Geometry: see drawing. Coordinates: mm, zero at the bounding-box minimum. Round coordinates to 2 decimals unless told otherwise and drop trailing zeros. Loops run counter-clockwise (first coordinate to the right, second up) from the corner with the lowest first, then second, coordinate; pieces in that order, holes last.
(1) Line query: line 1 (Y direction, x = 40, z = 2.25); line 2 (Y direction, x = 52, z = 0.35); line 3 (X direction, y = 85, z = 2.4). Output: solid intervals per line, ascending.
(2) Cut plane A-A, the plane y = 155. Output: boundary loops of the cut face in (x, z), and give its area (3 significant figures).
(3) Cut plane D-D, the plane y = 133.5. Output: boundary loops of the cut face in (x, z), and give its area (3 significant figures).
(4) Cut plane C-C, the plane z = 1.5. Output: boundary loops of the cut face in (x, y), and give its area (3 significant figures).
(5) Cut plane B-B, the plane x = 40. Output: boundary loops of the cut face in (y, z), and give its area (3 significant figures).
(6) First-contact query: pin 1 Ø10 at (x, y) = (21.5, 147.5) entering from -Z; pin 2 Ø2 at (x, z) = (14.5, 2.5) entering from +Y; pin 3 Ø1.5 at (y, z) = (37.5, 2.5) entering from +X; pin 4 Ø2.5 at (y, z) = (130.5, 3.5) entering from -X. Flat tips, straight axial feed; report the tip coordinate or a pass-through.
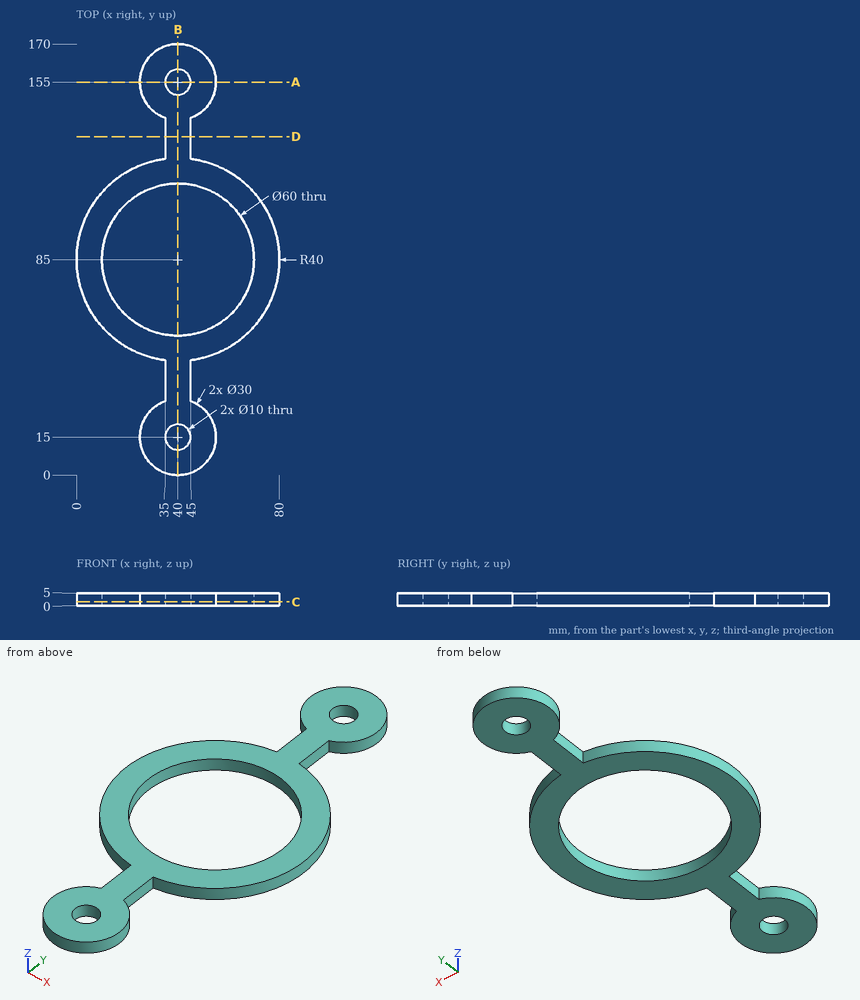
Reported:
1. line 1: y = 0 to 10, 20 to 55, 115 to 150, 160 to 170
1. line 2: y = 6 to 24, 46.84 to 57.5, 112.5 to 123.16, 146 to 164
1. line 3: x = 0 to 10, 70 to 80
2. outline: (25, 0) - (35, 0) - (35, 5) - (25, 5) - close; (45, 0) - (55, 0) - (55, 5) - (45, 5) - close
2. area: 100 mm2
3. outline: (35, 0) - (45, 0) - (45, 5) - (35, 5) - close
3. area: 50.0 mm2
4. outline: (35, 29.14) arc R15 ccw (long way) to (45, 29.14) - (45, 45.31) arc R40 ccw to (45, 124.69) - (45, 140.86) arc R15 ccw (long way) to (35, 140.86) - (35, 124.69) arc R40 ccw to (35, 45.31) - close; hole circle Ø60 at (40, 85); hole circle Ø10 at (40, 15); hole circle Ø10 at (40, 155)
4. area: 3,760 mm2
5. outline: (0, 0) - (10, 0) - (10, 5) - (0, 5) - close; (20, 0) - (55, 0) - (55, 5) - (20, 5) - close; (115, 0) - (150, 0) - (150, 5) - (115, 5) - close; (160, 0) - (170, 0) - (170, 5) - (160, 5) - close
5. area: 450 mm2
6. pin 1: stops at z = 0
6. pin 2: stops at y = 116.62
6. pin 3: stops at x = 45
6. pin 4: stops at x = 35
